Work out the finished part from the listing and answer in its coordinate system (mm). Face numbers are marked on the shaded views. Round coordinates to 2 decimals unless told otherwise and drop trailing zeros. Order: outer loops, then holes, each group sorted by start corner. A loop starts at its lowest first (then second) coordinate and runs counter-clockwise, first axis right, second up. Notation, with made-up numbers: (36.25, 21.5) -> (88.25, 21.5) arc R15 ccw to (88.25, 40.5) -> close; hole circle Ø3 at (37, -26). An arc over 180 degrees is marked (long way). Use one line per item in the form item = value.
Autodesk Inventor part; units mm, degrees
ref_plane "YZ Plane" through (0, 0, 0) normal (1, 0, 0) x (0, 1, 0)
ref_plane "XZ Plane" through (0, 0, 0) normal (0, 1, 0) x (-1, 0, 0)
ref_plane "XY Plane" through (0, 0, 0) normal (0, 0, 1) x (1, 0, 0)
sketch "Sketch1" plane through (0, 0, 0) normal (0, 1, 0) x (-1, 0, 0)
  line L0 (12.7, -12.7) -> (-12.7, -12.7)
  line L1 (-12.7, -12.7) -> (-12.7, 12.7)
  line L2 (-12.7, 12.7) -> (12.7, 12.7)
  line L3 (12.7, 12.7) -> (12.7, -12.7)
  line L4 (9.525, -9.525) -> (-9.525, -9.525)
  line L5 (-9.525, -9.525) -> (-9.525, 9.525)
  line L6 (-9.525, 9.525) -> (9.525, 9.525)
  line L7 (9.525, 9.525) -> (9.525, -9.525)
  point P0 (0, 0)
  point P1 (0, -9.525)
  point P2 (0, -12.7)
  point P3 (-9.525, 0)
  point P4 (-12.7, 0)
  dimension "d0" = 25.4
  dimension "d1" = 3.175
extrude "Extrusion1" add sketch "Sketch1" along normal blind 300
sketch "Sketch2" plane through (-12.7, 0, 12.7) normal (0, 0, 1) x (1, 0, 0)
  line L0 (0, 0) -> (0, 300) construction
  line L1 (0, 300) -> (25.4, 300) construction
  line L2 (25.4, 300) -> (25.4, 274.6) construction
  line L3 (25.4, 274.6) -> (0, 274.6) construction
  line L4 (0, 274.6) -> (0, 300) construction
  line L5 (25.4, 0) -> (25.4, 300) construction
  line L6 (8.4667, 291.5333) -> (16.9333, 291.5333) construction
  line L7 (16.9333, 291.5333) -> (16.9333, 283.0667) construction
  line L8 (16.9333, 283.0667) -> (8.4667, 283.0667) construction
  line L9 (8.4667, 283.0667) -> (8.4667, 291.5333) construction
  circle A0 centre (8.4667, 291.5333) radius 2.4257
  circle A1 centre (16.9333, 283.0667) radius 2.4257
  point P0 (12.7, 0)
  point P1 (12.7, 291.5333)
  point P2 (12.7, 300)
  point P3 (16.9333, 287.3)
  point P4 (25.4, 287.3)
  dimension "d4" = 8.4667
  dimension "d5" = 4.8514
sketch "Sketch3" plane through (-12.7, 0, -12.7) normal (-1, 0, 0) x (0, 0, 1)
  line L0 (0, 0) -> (0, 300) construction
  line L1 (0, 300) -> (25.4, 300) construction
  line L2 (25.4, 300) -> (25.4, 274.6) construction
  line L3 (25.4, 274.6) -> (0, 274.6) construction
  line L4 (0, 274.6) -> (0, 300) construction
  line L5 (8.4667, 291.5333) -> (16.9333, 291.5333) construction
  line L6 (16.9333, 291.5333) -> (16.9333, 283.0667) construction
  line L7 (16.9333, 283.0667) -> (8.4667, 283.0667) construction
  line L8 (8.4667, 283.0667) -> (8.4667, 291.5333) construction
  circle A0 centre (16.9333, 291.5333) radius 2.4257
  circle A1 centre (8.4667, 283.0667) radius 2.4257
  point P0 (12.7, 0)
  point P1 (16.9333, 287.3)
  point P2 (25.4, 287.3)
  point P3 (12.7, 283.0667)
  point P4 (12.7, 274.6)
  dimension "d6" = 25.4
  dimension "d7" = 8.4667
  dimension "d8" = 4.8514
extrude "Extrusion2" cut sketch "Sketch3" against normal blind 3.175
extrude "Extrusion3" cut sketch "Sketch2" against normal blind 3.175
properties part number "vertical"
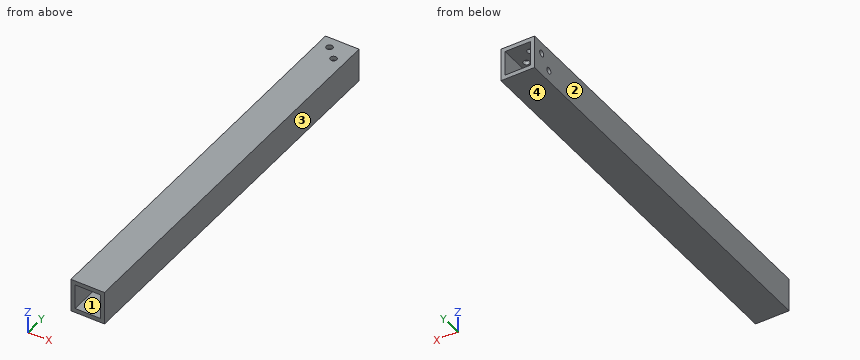
Item 1: Determine the mould class of the marked faces 1, 2, 3 and 4 for opening direction X: released by +X, released by -X, zero draft, split by the parting line, or undercut.
Findings:
face_1 = undercut
face_2 = released by -X
face_3 = released by +X
face_4 = zero draft
Item 2: A flat-ended cylindrical pin translates along its axis: P1, Ø4, axis at x = 4.23, y = 283.07, coming from the +Z side (3 decimals). Find the tip coordinate at first contact, or state that the pin passes through.
Findings:
P1 = -9.525
Item 3: Consider line 1 along X through (y, z) = (69, 6.5) (3 decimals); line 2 along Y through (x, z) = (-10.25, 4). Determine where each line is inside the solid, lowest interval first.
Findings:
line_1 = -12.7 to -9.525, 9.525 to 12.7
line_2 = 0 to 289.12, 293.95 to 300
Item 4: The part is cut by section A-A, the plane y = 21.5. Give the vertices of the cut face in (x, z) (3 decimals), and give its area (3 significant figures).
Findings:
outline = (-12.7, -12.7) -> (12.7, -12.7) -> (12.7, 12.7) -> (-12.7, 12.7) -> close; hole (-9.525, -9.525) -> (9.525, -9.525) -> (9.525, 9.525) -> (-9.525, 9.525) -> close
area = 282 mm^2
